from build123d import *

# Parameters (mm, degrees)
SKETCH1_R           = 11
BOSS_EXTRUDE1_DEPTH = 32
SKETCH2_R           = 5
BOSS_EXTRUDE2_DEPTH = 1.35
SKETCH3_R           = 3.5
BOSS_EXTRUDE4_DEPTH = 3.15
SKETCH4_R           = 2
BOSS_EXTRUDE5_DEPTH = 10.85
CUT_EXTRUDE1_START  = -9.3
CUT_EXTRUDE1_DEPTH  = 9.3


with BuildPart() as part:
    # Sketch1 → Boss-Extrude1 (new body)
    with BuildSketch(Plane.XY):
        Circle(SKETCH1_R)
    extrude(amount=BOSS_EXTRUDE1_DEPTH)

    # Sketch2 → Boss-Extrude2 (add)
    with BuildSketch(Plane.XY.offset(32)):
        with Locations(Location((0, 0, 0), (0, 0, 180))):
            Circle(SKETCH2_R)
    extrude(amount=BOSS_EXTRUDE2_DEPTH)

    # Sketch3 → Boss-Extrude4 (add)
    with BuildSketch(Plane.XY.offset(33.35)):
        Circle(SKETCH3_R)
    extrude(amount=BOSS_EXTRUDE4_DEPTH)

    # Sketch4 → Boss-Extrude5 (add)
    with BuildSketch(Plane.XY.offset(36.5)):
        Circle(SKETCH4_R)
    extrude(amount=BOSS_EXTRUDE5_DEPTH)

    # Sketch5 → Cut-Extrude1 (cut)
    with BuildSketch(Plane.XY.offset(47.35).offset(CUT_EXTRUDE1_START)):
        with BuildLine():
            Line((-0.338013059, 1.971229863), (-1.99802063, -0.088958203))
            ThreePointArc((-1.99802063, -0.088958203), (-1.557355793, 1.254847773), (-0.338013059, 1.971229863))
        make_face()
    extrude(amount=CUT_EXTRUDE1_DEPTH, mode=Mode.SUBTRACT)


solid = part.part
Source: CAD feature listing. Evaluate the final solid. Frame: model axes, mm. A direction names the side the tool comes from. Round coordinates to 2 decimals unless told otherwise and drop trailing zeros. Loops run counter-clockwise (first coordinate to the right, second up) from the corner with the lowest first, then second, coordinate; pieces in that order, holes last. Notation, with made-up numbers: M 59,48.25 L 118,48.25 A17 ccw 118,56.25 Z; hole C 61.25,77 d5. An arc over 180 degrees is marked long. Return JSON: item names as keys, results as strings. Group by question number.
1. Section query A-A on y = 0.75. Output: boundary loops of the cut face in (x, z).
2. Pin query (flat end, axial travel): pin 1 (8 mm diameter, centred on x = 8.5, z = 28.5, fed in from +Y); pin 2 (1.5 mm diameter, centred on x = -1.5, z = 10.5, fed in from -Y); pin 3 (2 mm diameter, centred on x = -1, y = 4, fed in from +Z). Return the tip coordinate at first contact, or that it passes through.
3. Section query C-C on x = -8. Output: boundary loops of the cut face in (y, z), and give its area (3 significant figures).
4. Reachability of faces 1 (the face through (-1.3, 1.1, 38.05)), 2 (the face through (-3.3, 2.2, 33.35)), 3 (the face through (-2.38, -10.74, 15.78)) from +Z, -Z, +X, -X, +Y, -Y: full face, straight path, thin tool, end or side. Return the list, or none.
5. Material intervals for line 1 along Z through (x, y) = (3, -9.25); line 2 along X through (y, z) = (0.25, 35); line 3 along X through (y, z) = (-0.5, 45.5), sorted ascending. Write a range as from..to.
6. Section query D-D on y = 3. Output: boundary loops of the cut face in (x, z).
7. Section query B-B on z = 39. Output: boundary loops of the cut face in (x, y), and give its area (3 significant figures).
Checks:
{
 "1": {"outline": "M -10.97,0 L 10.97,0 L 10.97,32 L 4.94,32 L 4.94,33.35 L 3.42,33.35 L 3.42,36.5 L 1.85,36.5 L 1.85,47.35 L -1.32,47.35 L -1.32,38.05 L -1.85,38.05 L -1.85,36.5 L -3.42,36.5 L -3.42,33.35 L -4.94,33.35 L -4.94,32 L -10.97,32 Z"},
 "2": {"pin 1": "stops at y = 10.04", "pin 2": "stops at y = -10.97", "pin 3": "stops at z = 36.5"},
 "3": {"outline": "M -7.55,0 L 7.55,0 L 7.55,32 L -7.55,32 Z", "area": "483 mm²"},
 "4": {"face 1": "+Z, -X, +Y", "face 2": "+Z", "face 3": "+Z, -Z"},
 "5": {"line 1": "z = 0..32", "line 2": "x = -3.49..3.49", "line 3": "x = -1.94..1.94"},
 "6": {"outline": "M -10.58,0 L 10.58,0 L 10.58,32 L 4,32 L 4,33.35 L 1.8,33.35 L 1.8,36.5 L -1.8,36.5 L -1.8,33.35 L -4,33.35 L -4,32 L -10.58,32 Z"},
 "7": {"outline": "M -2,-0.09 A2 ccw long -0.34,1.97 Z", "area": "11.7 mm²"}
}
